Can you work these out from the drawing? Everything is in mm from the part's minimum corner. A direction names the side the tool comes from. Round coordinates to 2 decimals unless told otherwise and drop trailing zeros. Write each loop counter-clockwise with the first axis right and the second up, starting at its lowest first coordinate (ties: lowest second). Pieces come first, ordered by that corner, then holes. Notation, with made-up numbers: (-29, -40) -> (2, -40) arc R31 cw to (2, -13) -> close; hole circle Ø7 at (-12.75, 6). An arc over 180 degrees is marked (long way). One line per question, with ' | ' between items. Start each with the question number.
1. Imagine slicing it at B-B, the plane x = 22.5. List the corners of the cut face in (y, z) for me.
2. Imagine slicing it at D-D, the plane x = 88. List the corners of the cut face in (y, z) for me.
3. For pin 1 Ø1 at (x, z) = (48.5, 9.5) entering from +Y; pin 2 Ø3 at (x, y) = (55.5, 5.5) entering from -Z; pin 3 Ø4.5 at (x, y) = (38, 6) entering from +Z, each with a flat end and sliding along its axis, tell me the tip position at first contact or that it passes through.
4. Imagine slicing it at A-A, the plane z = 52.5. List the corners of the cut face in (x, y) for me, and give its area (3 significant figures).
5. If I drill on line 1 along X through (y, z) = (11.2, 22.5); line 2 along X through (y, z) = (1.55, 5); line 3 along Y through (x, z) = (81, 30), over which ranges is the centre line in solid material (lowest first)? Write a range as [from, to].
6. For the marked faces 1, 2 and 3, which set-ups out of +Z, -Z, +X, -X, +Y, -Y let a thin tool reach every point of the face, with its end or its side?
7. Imagine slicing it at C-C, the plane x = 62. List the corners of the cut face in (y, z) for me.
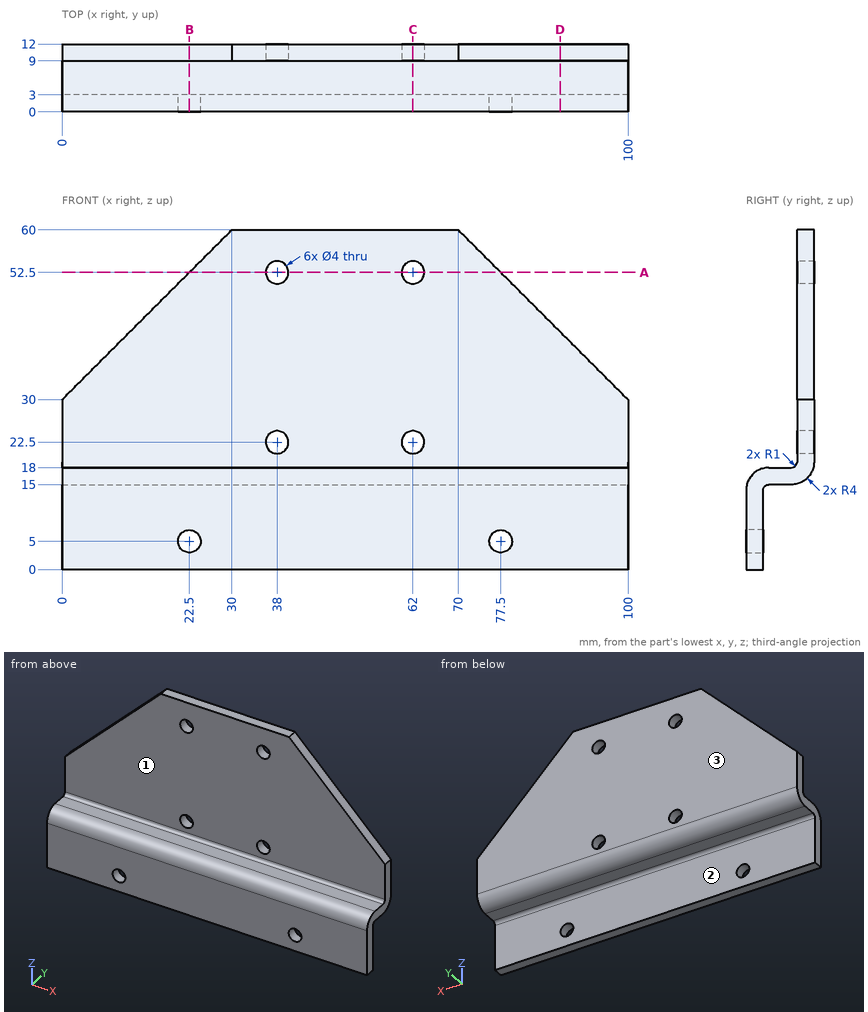
Geometry results:
1) outline: (0, 0) -> (3, 0) -> (3, 3) -> (0, 3) -> close; (0, 7) -> (3, 7) -> (3, 14) arc R1 cw to (4, 15) -> (8, 15) arc R4 ccw to (12, 19) -> (12, 52.5) -> (9, 52.5) -> (9, 19) arc R1 cw to (8, 18) -> (4, 18) arc R4 ccw to (0, 14) -> close
2) outline: (0, 0) -> (3, 0) -> (3, 14) arc R1 cw to (4, 15) -> (8, 15) arc R4 ccw to (12, 19) -> (12, 42) -> (9, 42) -> (9, 19) arc R1 cw to (8, 18) -> (4, 18) arc R4 ccw to (0, 14) -> close
3) pin 1: stops at y = 3 | pin 2: stops at z = 15 | pin 3: stops at z = 18.03
4) outline: (22.5, 9) -> (36, 9) -> (36, 12) -> (22.5, 12) -> close; (40, 9) -> (60, 9) -> (60, 12) -> (40, 12) -> close; (64, 9) -> (77.5, 9) -> (77.5, 12) -> (64, 12) -> close | area: 141 mm2
5) line 1: x = [0, 36], [40, 60], [64, 100] | line 2: x = [0, 20.5], [24.5, 75.5], [79.5, 100] | line 3: y = [9, 12]
6) face 1: +Z, +X, -X, -Y | face 2: -Z, +X, -X, +Y | face 3: +Z, -Z, +X, -X, +Y
7) outline: (0, 0) -> (3, 0) -> (3, 14) arc R1 cw to (4, 15) -> (8, 15) arc R4 ccw to (12, 19) -> (12, 20.5) -> (9, 20.5) -> (9, 19) arc R1 cw to (8, 18) -> (4, 18) arc R4 ccw to (0, 14) -> close; (9, 24.5) -> (12, 24.5) -> (12, 50.5) -> (9, 50.5) -> close; (9, 54.5) -> (12, 54.5) -> (12, 60) -> (9, 60) -> close
